```python
from build123d import *

# Parameters (mm, degrees)
F0_W      = 50
F0_H      = 280
F1_DEPTH  = 3
F2_W      = 3
F2_H      = 20
F3_DEPTH  = 25
F4_W      = 7.5
F4_H      = 3
F5_DEPTH  = 25
F6_W      = 50
F6_H      = 30.25
F7_DEPTH  = 3
F8_W      = 3
F8_H      = 10
F9_DEPTH  = 25
F10_W     = 7.5
F10_H     = 3
F11_DEPTH = 25


with BuildPart() as f1:
    # F0 (on Top) → F1 (new body)
    with BuildSketch(Plane.XY):
        Rectangle(F0_W, F0_H)
    extrude(amount=F1_DEPTH)

    # F2 (on face) → F3 (cut)
    with BuildSketch(Plane.XY.offset(3)):
        with Locations((3, 120)):
            Rectangle(F2_W, F2_H)
        with Locations((3, 80)):
            Rectangle(F2_W, F2_H)
        with Locations((3, 40)):
            Rectangle(F2_W, F2_H)
        with Locations((3, 0)):
            Rectangle(F2_W, F2_H)
        with Locations((3, -40)):
            Rectangle(F2_W, F2_H)
        with Locations((3, -80)):
            Rectangle(F2_W, F2_H)
        with Locations((3, -120)):
            Rectangle(F2_W, F2_H)
        with Locations((-3, 120)):
            Rectangle(F2_W, F2_H)
        with Locations((-3, 80)):
            Rectangle(F2_W, F2_H)
        with Locations((-3, 40)):
            Rectangle(F2_W, F2_H)
        with Locations((-3, 0)):
            Rectangle(F2_W, F2_H)
        with Locations((-3, -40)):
            Rectangle(F2_W, F2_H)
        with Locations((-3, -80)):
            Rectangle(F2_W, F2_H)
        with Locations((-3, -120)):
            Rectangle(F2_W, F2_H)
    extrude(amount=-F3_DEPTH, mode=Mode.SUBTRACT)

    # F4 (on face) → F5 (cut)
    with BuildSketch(Plane.XY.offset(3)):
        with Locations((15.75, 120)):
            Rectangle(F4_W, F4_H)
        with Locations((15.75, 80)):
            Rectangle(F4_W, F4_H)
        with Locations((15.75, 40)):
            Rectangle(F4_W, F4_H)
        with Locations((15.75, 0)):
            Rectangle(F4_W, F4_H)
        with Locations((15.75, -40)):
            Rectangle(F4_W, F4_H)
        with Locations((15.75, -80)):
            Rectangle(F4_W, F4_H)
        with Locations((15.75, -120)):
            Rectangle(F4_W, F4_H)
        with Locations((-15.75, 120)):
            Rectangle(F4_W, F4_H)
        with Locations((-15.75, -80)):
            Rectangle(F4_W, F4_H)
        with Locations((-15.75, 40)):
            Rectangle(F4_W, F4_H)
        with Locations((-15.75, 80)):
            Rectangle(F4_W, F4_H)
        with Locations((-15.75, -40)):
            Rectangle(F4_W, F4_H)
        with Locations((-15.75, -120)):
            Rectangle(F4_W, F4_H)
        with Locations((-15.75, 0)):
            Rectangle(F4_W, F4_H)
    extrude(amount=-F5_DEPTH, mode=Mode.SUBTRACT)

    # F6 (on face) → F7 (join)
    with BuildSketch(Plane.XY.offset(3)):
        with Locations((0, 155.125)):
            Rectangle(F6_W, F6_H)
        with Locations((0, -155.125)):
            Rectangle(F6_W, F6_H)
    extrude(amount=-F7_DEPTH)

    # F8 (on face) → F9 (cut)
    with BuildSketch(Plane.XY.offset(3)):
        with Locations((-3, 155)):
            Rectangle(F8_W, F8_H)
        with Locations((3, 155)):
            Rectangle(F8_W, F8_H)
        with Locations((3, -155)):
            Rectangle(F8_W, F8_H)
        with Locations((-3, -155)):
            Rectangle(F8_W, F8_H)
    extrude(amount=-F9_DEPTH, mode=Mode.SUBTRACT)

    # F10 (on face) → F11 (cut)
    with BuildSketch(Plane.XY.offset(3)):
        with Locations((-15.75, -155)):
            Rectangle(F10_W, F10_H)
        with Locations((15.75, -155)):
            Rectangle(F10_W, F10_H)
        with Locations((-15.75, 155)):
            Rectangle(F10_W, F10_H)
        with Locations((15.75, 155)):
            Rectangle(F10_W, F10_H)
    extrude(amount=-F11_DEPTH, mode=Mode.SUBTRACT)


solid = f1.part
```
Source: CAD feature listing. Evaluate the final solid. Frame: model axes, mm. Give positions to 0.01 mm unless a question says otherwise; leave off trailing zeros.
(1) Material intervals for line 1 along X through (y, z) = (5.5, 2.15), sorted ascending.
(2) Contact query for a flat-ended pin moving along its axis: P1, Ø5, axis at x = -18, y = -40, coming from the -Z side. Output: stop coordinate, or through.
(3) Section query A-A (z = 1.55). State how many separate pieces and enclosed holes the cut face has, plus the area to 3 significant figures.
Outcome:
1. line 1: x = -25 to -4.5, -1.5 to 1.5, 4.5 to 25
2. P1: stops at z = 0
3. separate pieces: 1
3. enclosed holes: 36
3. area: 15,700 mm2
